```python
from build123d import *

# Parameters (mm, degrees)
EXTRUDE_2_DEPTH     = 4
EXTRUDE_3_DEPTH     = 4
SKETCH_3_R          = 0.25
CUT_EXTRUDE_1_DEPTH = 4


with BuildPart() as part:
    # 草图1 → 凸台-拉伸2 (new body)
    with BuildSketch(Plane(origin=(0, 0, 0), x_dir=(0, 0, -1), z_dir=(1, 0, 0))):
        Polygon((-4.326044833, 1.768613288), (5.673955167, 1.768613288), (5.673955167, 0.768613288), (-4.04400015, 0.768613288), (-13.803521761, -5.212415113), (-14.326044833, -4.359789967), align=None)
    extrude(amount=EXTRUDE_2_DEPTH)

    # 草图2 → 凸台-拉伸3 (add)
    with BuildSketch(Plane(origin=(4, 0, 0), x_dir=(0, 0, -1), z_dir=(1, 0, 0))):
        with BuildLine():
            Line((5.673955167, 0.768613288), (5.673955167, 1.768613288))
            ThreePointArc((5.673955167, 1.768613288), (6.173955167, 1.268613288), (5.673955167, 0.768613288))
        make_face()
        with BuildLine():
            Line((-14.326044833, -4.359789967), (-13.803521761, -5.212415113))
            ThreePointArc((-13.803521761, -5.212415113), (-14.49109587, -5.047364076), (-14.326044833, -4.359789967))
        make_face()
    extrude(amount=-EXTRUDE_3_DEPTH)

    # 草图3 → 切除-拉伸1 (cut)
    with BuildSketch(Plane(origin=(4, 0, 0), x_dir=(0, 0, -1), z_dir=(1, 0, 0))):
        with Locations((-14.064783297, -4.78610254)):
            Circle(SKETCH_3_R)
        with Locations((5.673955167, 1.268613288)):
            Circle(SKETCH_3_R)
    extrude(amount=-CUT_EXTRUDE_1_DEPTH, mode=Mode.SUBTRACT)


solid = part.part
```
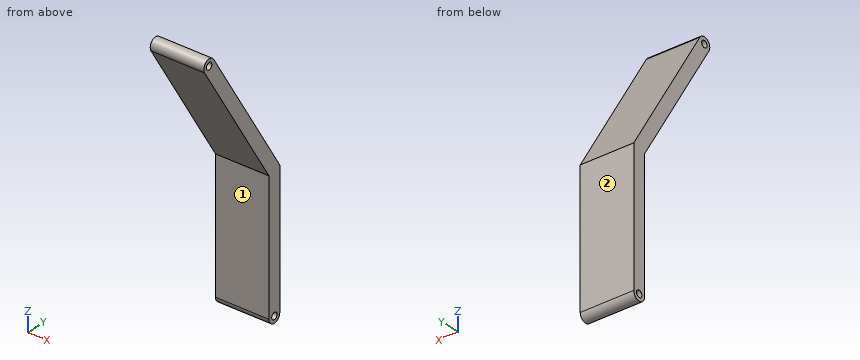
Could you check a few things on this model? Use its own coordinates, in mm. Face numbers are marked on the shaded views. A direction names the side the tool comes from. Give positions to 0.01 mm unless a question says otherwise; leave off trailing zeros. Order: outer loops, then holes, each group sorted by start corner. A loop starts at its lowest first (then second) coordinate and runs counter-clockwise, first axis right, second up.
Q1. Suppose I cut it at A-A, the plane x = 3.05. Write out the boundary of the cut face in (y, z).
Q2. Suppose I cut it at B-B, the plane z = -2. Write out the boundary of the cut face in (x, y).
Q3. If I drill on line 1 along Y through (x, z) = (0.7, -3.25); line 2 along Z through (x, y) = (3.3, 1.25); line 3 along Z through (x, y) = (2.25, -3), over which ranges is the centre line in solid material (lowest first)?
Q4. For the marked faces 1 and 2, which set-ups out of +Z, -Z, +X, -X, +Y, -Y let a thin tool reach every point of the face, with its end or its side?
Q5. Suppose I cut it at C-C, the plane y = -1. Write out the boundary of the cut face in (x, z).
Q6. I'm going to push flat-ended pins straight in: P1, Ø1, axis at x = 2, z = 3, coming from the -Y side; P2, Ø1.5, axis at y = -2.5, z = 5.5, coming from the +X side. Where does each tip first touch, or does it pass through?
Solution:
1. outline: (-5.21, 13.8) - (0.77, 4.04) - (0.77, -5.67) arc R0.5 ccw to (1.77, -5.67) - (1.77, 4.33) - (-4.36, 14.33) arc R0.5 ccw to start; hole circle Ø0.5 at (-4.79, 14.06); hole circle Ø0.5 at (1.27, -5.67)
2. outline: (0, 0.77) - (4, 0.77) - (4, 1.77) - (0, 1.77) - close
3. line 1: y = 0.77 to 1.77
3. line 2: z = -6.17 to -5.92, -5.42 to 5.17
3. line 3: z = 10.19 to 12.11
4. face 1: -Z, +X, -X, -Y
4. face 2: +Z, -Z, +X, -X, +Y
5. outline: (0, 6.93) - (4, 6.93) - (4, 8.84) - (0, 8.84) - close
6. P1: stops at y = 0.77
6. P2: passes through
